Design review of the part built by this model. Coordinates are the model's own, in mm. Face numbers are marked on the shaded views. A direction names the side the tool comes from. Coordinates: 2 decimals unless noted, no trailing zeros. Write each loop counter-clockwise with the first axis right and the second up, starting at its lowest first coordinate (ties: lowest second). Pieces come first, ordered by that corner, then holes. Notation, with made-up numbers: (85, 13) - (142, 13) arc R18 cw to (142, 17) - close; hole circle Ø11 at (84.5, 54.25). An arc over 180 degrees is marked (long way). Answer as a JSON object with one key per item and string values.
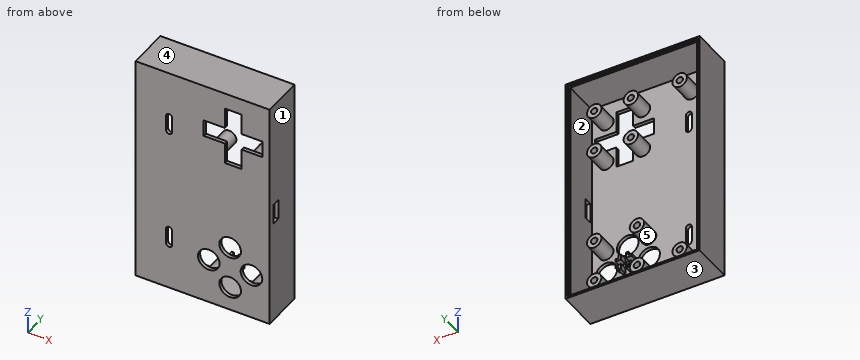
Autodesk Inventor part; units mm, degrees
ref_plane "YZ Plane" through (0, 0, 0) normal (1, 0, 0) x (0, 1, 0)
ref_plane "XZ Plane" through (0, 0, 0) normal (0, 1, 0) x (-1, 0, 0)
ref_plane "XY Plane" through (0, 0, 0) normal (0, 0, 1) x (1, 0, 0)
sketch "Skizze1" plane through (0, 0, 0) normal (0, 1, 0) x (-1, 0, 0)
  line L0 (0, 0) -> (55.8, 0)
  line L1 (55.8, 0) -> (55.8, -96.44)
  line L2 (55.8, -96.44) -> (0, -96.44)
  line L3 (0, -96.44) -> (0, 0)
  dimension "d0" = 96.44
  dimension "d1" = 55.8
extrude "Extrusion1" add sketch "Skizze1" against normal blind 1.5
sketch "Skizze2" plane through (0, 0, 0) normal (0, 1, 0) x (1, 0, 0)
  line L0 (0, 0) -> (-55.8, 0)
  line L1 (-55.8, 0) -> (-55.8, 96.44)
  line L2 (0, 0) -> (-55.8, 0)
  line L3 (-55.8, 0) -> (-55.8, 96.44)
  line L4 (-55.8, 96.44) -> (0, 96.44)
  line L5 (0, 96.44) -> (0, 0)
  line L6 (-1.5, 1.5) -> (-54.3, 1.5)
  line L7 (-54.3, 1.5) -> (-54.3, 94.94)
  line L8 (-54.3, 94.94) -> (-1.5, 94.94)
  line L9 (-1.5, 94.94) -> (-1.5, 1.5)
  dimension "d4" = 1.5
extrude "Extrusion2" add sketch "Skizze2" along normal blind 15.75
sketch "Skizze4" plane through (0, 0, 0) normal (0, 1, 0) x (1, 0, 0)
  circle A0 centre (-22.82, 10.12) radius 3
  circle A1 centre (-22.82, 27.9) radius 3
  circle A2 centre (-7.58, 27.9) radius 3
  circle A3 centre (-7.58, 10.12) radius 3
  line L0 (-18.7, 6.76) -> (-18.7, 15.51)
  line L1 (-27.45, 22.51) -> (-18.7, 22.51)
  line L2 (-11.7, 15.51) -> (-11.7, 6.76)
  line L3 (-11.7, 31.26) -> (-11.7, 22.51)
  circle A4 centre (-22.82, 10.12) radius 1.3
  circle A5 centre (-22.82, 27.9) radius 1.3
  circle A6 centre (-7.58, 27.9) radius 1.3
  circle A7 centre (-7.58, 10.12) radius 1.3
  line L4 (-1.5, 1.5) -> (-54.3, 1.5)
  line L5 (-27.45, 22.51) -> (-27.45, 15.51)
  line L6 (-27.45, 15.51) -> (-18.7, 15.51)
  line L7 (-11.7, 22.51) -> (-2.95, 22.51)
  line L8 (-2.95, 22.51) -> (-2.95, 15.51)
  line L9 (-2.95, 15.51) -> (-11.7, 15.51)
  line L10 (-11.7, 6.76) -> (-18.7, 6.76)
  line L11 (-18.7, 22.51) -> (-18.7, 31.26)
  line L12 (-18.7, 31.26) -> (-11.7, 31.26)
  line L13 (-54.3, 1.5) -> (-54.3, 94.94)
  line L14 (-1.5, 94.94) -> (-1.5, 1.5)
  point P0 (0, 0)
  dimension "d13" = 4.12
  dimension "d15" = 4.12
  dimension "d16" = 4.12
  dimension "d17" = 6
  dimension "d18" = 6
  dimension "d19" = 6
  dimension "d20" = 6
  dimension "d21" = 2.6
  dimension "d22" = 2.6
  dimension "d23" = 2.6
  dimension "d24" = 2.6
  dimension "d25" = 17.78
  dimension "d29" = 17.78
  dimension "d30" = 15.24
  dimension "d31" = 15.24
  dimension "d32" = 4.12
  dimension "d33" = 7
  dimension "d34" = 7
  dimension "d35" = 7
  dimension "d36" = 7
  dimension "d37" = 8.75
  dimension "d38" = 8.75
  dimension "d39" = 8.75
  dimension "d40" = 8.75
  dimension "d41" = 8.75
  dimension "d42" = 8.75
  dimension "d43" = 8.75
  dimension "d44" = 8.75
  dimension "d45" = 5.39
  dimension "d46" = 8.62
  dimension "d48" = 5.39
  dimension "d147" = 6.08
extrude "Extrusion3" cut sketch "Skizze4" against normal blind 15 contours L0 L6 L5 L1 L11 L12 L3 L7 L8 L9 L2 L10
extrude "Extrusion4" add sketch "Skizze4" along normal blind 8.5 contours A0 | A1 | A2 | A3
sketch "Skizze5" plane through (0, 0, 0) normal (0, 1, 0) x (1, 0, 0)
  line L0 (-54.3, 1.5) -> (-54.3, 94.94)
  line L1 (-54.3, 94.94) -> (-1.5, 94.94)
  circle A0 centre (-25.36, 77.43) radius 4.5
  circle A1 centre (-7.58, 77.43) radius 4.5
  circle A2 centre (-16.47, 86.32) radius 4.5
  circle A3 centre (-16.47, 68.54) radius 4.5
  circle A4 centre (-25.36, 68.54) radius 3
  circle A5 centre (-25.36, 68.54) radius 1.35
  circle A6 centre (-25.36, 86.32) radius 3
  circle A7 centre (-25.36, 86.32) radius 1.35
  circle A8 centre (-7.58, 86.32) radius 3
  circle A9 centre (-7.58, 86.32) radius 1.35
  circle A10 centre (-7.58, 68.54) radius 3
  circle A11 centre (-7.58, 68.54) radius 1.35
  line L2 (-18.47, 74.04) -> (-18.47, 75.43)
  line L3 (-18.47, 75.43) -> (-19.86, 75.43)
  line L4 (-19.86, 75.43) -> (-19.86, 76.43)
  line L5 (-19.86, 76.43) -> (-17.47, 76.43)
  line L6 (-17.47, 76.43) -> (-17.47, 74.04)
  line L7 (-17.47, 74.04) -> (-18.47, 74.04)
  line L8 (-15.47, 74.04) -> (-15.47, 76.43)
  line L9 (-15.47, 76.43) -> (-13.08, 76.43)
  line L10 (-13.08, 76.43) -> (-13.08, 75.43)
  line L11 (-13.08, 75.43) -> (-14.47, 75.43)
  line L12 (-14.47, 75.43) -> (-14.47, 74.04)
  line L13 (-14.47, 74.04) -> (-15.47, 74.04)
  line L14 (-17.47, 78.43) -> (-17.47, 80.82)
  line L15 (-17.47, 80.82) -> (-18.47, 80.82)
  line L16 (-18.47, 80.82) -> (-18.47, 79.43)
  line L17 (-18.47, 79.43) -> (-19.86, 79.43)
  line L18 (-19.86, 79.43) -> (-19.86, 78.43)
  line L19 (-19.86, 78.43) -> (-17.47, 78.43)
  line L20 (-15.47, 78.43) -> (-13.08, 78.43)
  line L21 (-13.08, 78.43) -> (-13.08, 79.43)
  line L22 (-13.08, 79.43) -> (-14.47, 79.43)
  line L23 (-14.47, 79.43) -> (-14.47, 80.82)
  line L24 (-14.47, 80.82) -> (-15.47, 80.82)
  line L25 (-15.47, 80.82) -> (-15.47, 78.43)
  line L26 (-1.5, 94.94) -> (-1.5, 1.5)
  point P0 (0, 0)
  dimension "d92" = 9
  dimension "d93" = 9
  dimension "d94" = 9
  dimension "d95" = 9
  dimension "d96" = 8.62
  dimension "d98" = 8.89
  dimension "d99" = 8.89
  dimension "d100" = 8.89
  dimension "d101" = 8.89
  dimension "d102" = 6
  dimension "d103" = 2.7
  dimension "d104" = 6
  dimension "d105" = 2.7
  dimension "d106" = 6
  dimension "d107" = 2.7
  dimension "d108" = 6
  dimension "d109" = 2.7
  dimension "d110" = 8.89
  dimension "d115" = 2
  dimension "d116" = 1
  dimension "d117" = 1
  dimension "d118" = 1
  dimension "d121" = 1
  dimension "d129" = 1
  dimension "d130" = 1
  dimension "d131" = 1
  dimension "d134" = 5.5
  dimension "d135" = 5.5
  dimension "d136" = 5.5
  dimension "d137" = 5.5
  dimension "d138" = 2
  dimension "d139" = 2
  dimension "d140" = 2.39
  dimension "d141" = 2.39
  dimension "d142" = 2.39
  dimension "d143" = 1
  dimension "d144" = 2.39
  dimension "d148" = 6.08
extrude "Extrusion5" cut sketch "Skizze5" against normal blind 15 contours A0 | A1 | A2 | A3
extrude "Extrusion6" add sketch "Skizze5" along normal blind 8.5 contours A4 | A6 | A8 | A10
extrude "Extrusion7" add sketch "Skizze5" along normal blind 3 contours L2 L3 L4 L5 L6 L7 | L8 L9 L10 L11 L12 L13 | L19 L18 L17 L16 L15 L14 | L25 L24 L23 L22 L21 L20
sketch "Skizze6" plane through (0, 0, 0) normal (0, 1, 0) x (1, 0, 0)
  line L0 (-43.12, 19.57) -> (-43.12, 26.07)
  line L1 (-40.62, 26.07) -> (-40.62, 19.57)
  arc A0 (-43.12, 19.57) -> (-40.62, 19.57) centre (-41.87, 19.57) ccw
  arc A1 (-40.62, 26.07) -> (-43.12, 26.07) centre (-41.87, 26.07) ccw
  circle A2 centre (-22.82, 27.9) radius 1.3
  line L2 (-43.12, 70.37) -> (-43.12, 76.87)
  line L3 (-40.62, 76.87) -> (-40.62, 70.37)
  arc A3 (-43.12, 70.37) -> (-40.62, 70.37) centre (-41.87, 70.37) ccw
  arc A4 (-40.62, 76.87) -> (-43.12, 76.87) centre (-41.87, 76.87) ccw
  circle A5 centre (-25.36, 86.32) radius 1.35
  circle A6 centre (-25.36, 68.54) radius 1.35
  point P0 (0, 0)
  dimension "d149" = 6.5
  dimension "d150" = 2.5
  dimension "d151" = 19.05
  dimension "d152" = 1.83
  dimension "d153" = 6.5
  dimension "d154" = 2.5
  dimension "d156" = 16.51
  dimension "d157" = 1.83
extrude "Extrusion8" cut sketch "Skizze6" against normal blind 3 contours L0 A1 L1 A0 | L2 A4 L3 A3
sketch "Skizze7" plane through (0, 0, 0) normal (0, 1, 0) x (1, 0, 0)
  circle A0 centre (-43.14, 86.32) radius 3
  circle A1 centre (-43.14, 10.12) radius 3
  circle A2 centre (-43.14, 86.32) radius 1.35
  circle A3 centre (-43.14, 10.12) radius 1.35
  line L0 (-1.5, 1.5) -> (-54.3, 1.5)
  line L1 (-1.5, 94.94) -> (-1.5, 1.5)
  circle A4 centre (-25.36, 86.32) radius 1.35
  circle A5 centre (-22.82, 10.12) radius 1.3
  point P0 (0, 0)
  dimension "d160" = 6
  dimension "d161" = 6
  dimension "d162" = 2.7
  dimension "d163" = 2.7
  dimension "d167" = 0
  dimension "d168" = 0
  dimension "d169" = 17.78
  dimension "d170" = 20.32
extrude "Extrusion9" add sketch "Skizze7" along normal blind 8.5 contours A0 | A1
sketch "Skizze9" plane through (0, -1.5, 0) normal (1, 0, 0) x (0, 0, -1)
  line L0 (44.47, 6) -> (52.97, 6)
  line L1 (52.97, 6) -> (52.97, 2.5)
  line L2 (52.97, 2.5) -> (44.47, 2.5)
  line L3 (44.47, 2.5) -> (44.47, 6)
  line L4 (1.5, 1.5) -> (94.94, 1.5)
  line L5 (0, 0) -> (0, 17.25)
  point P0 (0, 1.5)
  dimension "d173" = 4.5
  dimension "d174" = 1
  dimension "d175" = 8.5
  dimension "d177" = 44.47
extrude "Extrusion10" cut sketch "Skizze9" against normal blind 8.5
sketch "Skizze14" plane through (0, 15.75, 0) normal (0, 1, 0) x (1, 0, 0)
  line L0 (-1.5, 1.5) -> (-54.3, 1.5)
  line L1 (-1.5, 1.5) -> (-1.5, 94.94)
  line L2 (-54.3, 1.5) -> (-1.5, 1.5)
  line L3 (-1.5, 1.5) -> (-1.5, 94.94)
  line L4 (-1.5, 94.94) -> (-54.3, 94.94)
  line L5 (-54.3, 94.94) -> (-54.3, 1.5)
  line L6 (-55.05, 95.69) -> (-0.75, 95.69)
  line L7 (-0.75, 95.69) -> (-0.75, 0.75)
  line L8 (-0.75, 0.75) -> (-55.05, 0.75)
  line L9 (-55.05, 0.75) -> (-55.05, 95.69)
  point P0 (0, 0)
  dimension "d180" = 0.75
extrude "Extrusion11" cut sketch "Skizze14" against normal blind 0.75
properties part number "Front"
(1) The part is to be moulded in two halves that separate along X. For the marked faces 1, 2 and 3, say which applies: pulls with the +X half, pulls with the -X half, needs draft (parallel to the pull), parting line crosses it, or undercut.
Solved:
{"face 1": "pulls with the +X half", "face 2": "undercut", "face 3": "needs draft"}
(2) Take a section at C-C, the plane y = 13.5. Write out the cut boundary in (x, z), and give its area (3 significant figures).
Solved:
{"outline": "(-55.8, -96.44) - (0, -96.44) - (0, 0) - (-55.8, 0) - close; hole (-54.3, -94.94) - (-1.5, -94.94) - (-1.5, -1.5) - (-54.3, -1.5) - close", "area": "448 mm^2"}
(3) Take a section at B-B, the plane z = -35. Write out the cut boundary in (x, y).
Solved:
{"outline": "(-55.8, -1.5) - (0, -1.5) - (0, 15.75) - (-0.75, 15.75) - (-0.75, 15) - (-1.5, 15) - (-1.5, 0) - (-54.3, 0) - (-54.3, 15) - (-55.05, 15) - (-55.05, 15.75) - (-55.8, 15.75) - close"}
(4) Tool access review of the marked faces 4 and 5: name each direction out of +Z, -Z, +X, -X, +Y, -Y from which nothing blocks a thin tool from reaching the whole face with its end or side.
Solved:
{"face 4": "+Z, +X, -X, +Y, -Y", "face 5": "+Y"}
(5) Take a section at A-A, the plane y = 7. Give the number of separate pieces and of enclosed holes in the cut face, and give its area (3 significant figures).
Solved:
{"separate pieces": "11", "enclosed holes": "11", "area": "675 mm^2"}
(6) To check wall thickness, follow line 1 (X direction, y = 3.75, z = -68.54); line 2 (Z direction, x = -43.14, y = 4.25); line 3 (X direction, y = 6.75, z = -27.9). State the ranges of each line that lie inside material, in increasing order. Write a range as from..to.
Solved:
{"line 1": "x = -55.8..-54.3, -28.36..-26.71, -24.01..-22.36, -10.58..-8.93, -6.23..-4.58, -1.5..0", "line 2": "z = -96.44..-94.94, -89.32..-87.67, -84.97..-83.32, -13.12..-11.47, -8.77..-7.12, -1.5..0", "line 3": "x = -55.8..-54.3, -25.82..-24.12, -21.52..-19.82, -10.58..-8.88, -6.28..-4.58, -1.5..0"}
(7) For pin 1 (1.9 mm diameter, centred on x = -14.5, z = -79.5, fed in from +Y); pin 2 (3 mm diameter, centred on x = -8, z = -86.5, fed in from +Y); pin 3 (3 mm diameter, centred on x = -22.5, z = -38, fed in from +Y), all flat-tipped, find the tip position at first contact; note any pin that passes through.
Solved:
{"pin 1": "stops at y = 3", "pin 2": "stops at y = 8.5", "pin 3": "stops at y = 0"}
